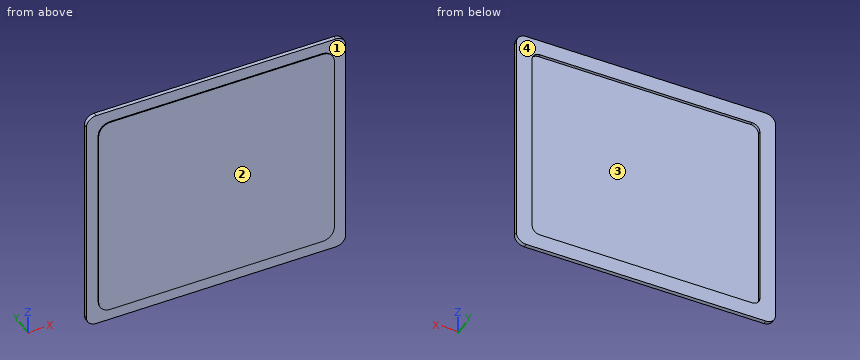
from build123d import *

# Parameters (mm, degrees)
RESSALTO_EXTRUS_O2_DEPTH = 10
RESSALTO_EXTRUS_O3_DEPTH = 2.5


with BuildPart() as part:
    # Esboço1 → Ressalto-extrusão2 (new body)
    with BuildSketch(Plane(origin=(0, 0, 0), x_dir=(1, 0, 0), z_dir=(0, 1, 0))):
        with BuildLine():
            Line((-305, -300), (305, -300))
            ThreePointArc((305, -300), (322.67766953, -292.67766953), (330, -275))
            Line((330, -275), (330, 275))
            ThreePointArc((330, 275), (322.67766953, 292.67766953), (305, 300))
            Line((305, 300), (-305, 300))
            ThreePointArc((-305, 300), (-322.67766953, 292.67766953), (-330, 275))
            Line((-330, 275), (-330, -275))
            ThreePointArc((-330, -275), (-322.67766953, -292.67766953), (-305, -300))
        make_face()
        with BuildLine():
            Line((270, -260), (-270, -260))
            ThreePointArc((-270, -260), (-284.142135624, -254.142135624), (-290, -240))
            Line((-290, -240), (-290, 240))
            ThreePointArc((-290, 240), (-284.142135624, 254.142135624), (-270, 260))
            Line((-270, 260), (270, 260))
            ThreePointArc((270, 260), (284.142135624, 254.142135624), (290, 240))
            Line((290, 240), (290, -240))
            ThreePointArc((290, -240), (284.142135624, -254.142135624), (270, -260))
        make_face(mode=Mode.SUBTRACT)
    extrude(amount=RESSALTO_EXTRUS_O2_DEPTH)

    # Esboço2 → Ressalto-extrusão3 (add, symmetric)
    with BuildSketch(Plane(origin=(0, 0, 0), x_dir=(1, 0, 0), z_dir=(0, 1, 0))):
        with BuildLine():
            Line((300, -240), (300, 240))
            ThreePointArc((300, 240), (291.213203436, 261.213203436), (270, 270))
            Line((270, 270), (-270, 270))
            ThreePointArc((-270, 270), (-291.213203436, 261.213203436), (-300, 240))
            Line((-300, 240), (-300, -240))
            ThreePointArc((-300, -240), (-291.213203436, -261.213203436), (-270, -270))
            Line((-270, -270), (270, -270))
            ThreePointArc((270, -270), (291.213203436, -261.213203436), (300, -240))
        make_face()
    extrude(amount=RESSALTO_EXTRUS_O3_DEPTH, both=True)


solid = part.part
For this review, take the finished solid that the model builds, in its own axes (mm). Face numbers are marked on the shaded views. A direction names the side the tool comes from. Coordinates: 2 decimals unless noted, no trailing zeros. Loops run counter-clockwise (first coordinate to the right, second up) from the corner with the lowest first, then second, coordinate; pieces in that order, holes last. Notation, with made-up numbers: (-32, 62.5) - (25, 62.5) arc R35 ccw to (25, 94.5) - close; hole circle Ø11 at (56.5, -38.75). An arc over 180 degrees is marked (long way). Use a Markdown table: item, result. Add a question column.
Item 1: Tool access review of the marked faces 1 and 2: name each direction out of +Z, -Z, +X, -X, +Y, -Y from which nothing blocks a thin tool from reaching the whole face with its end or side.
Item 2: We need section B-B (x = -45.5). Give the boundary of the cut face in (y, z).
Item 3: For line 1 (X direction, y = 5.25, z = -145); line 2 (Z direction, x = 10, y = 4.5); line 3 (Y direction, x = 5, z = -191.5), list the stretches that pass through material, from the lowest coordinate up.
Item 4: We need section C-C (z = -108). Give the boundary of the cut face in (x, y), and give its area (3 significant figures).
Item 5: Mouldability with a two-part tool opening along X and no side actions: class the marked faces 3 and 4 as pulls with the +X half, pulls with the -X half, needs draft (parallel to the pull), parting line crosses it, or undercut.
Item 6: We need section A-A (y = 6). Give the boundary of the cut face in (x, z).
Item 7: Insertion check: pin 1 Ø0.8 at (x, y) = (-117, -0.5) entering from +Z; pin 2 Ø6 at (x, z) = (-134.5, -118) entering from +Y; pin 3 Ø0.8 at (y, z) = (-1.5, 104.5) entering from -X; pin 4 Ø2 at (x, y) = (-37.5, -0.5) entering from -Z. Each pin has a flat end and moves straight along its axis. Give the tip position at first contact, or say it passes through.
Results list:
| question | item | result |
|---|---|---|
| 1 | face 1 | -Y |
| 1 | face 2 | +Z, -Z, +X, -X, -Y |
| 2 | outline | (-2.5, -270) - (0, -270) - (0, -300) - (10, -300) - (10, -260) - (2.5, -260) - (2.5, 260) - (10, 260) - (10, 300) - (0, 300) - (0, 270) - (-2.5, 270) - close |
| 3 | line 1 | x = -330 to -290, 290 to 330 |
| 3 | line 2 | z = -300 to -260, 260 to 300 |
| 3 | line 3 | y = -2.5 to 2.5 |
| 4 | outline | (-330, 0) - (-300, 0) - (-300, -2.5) - (300, -2.5) - (300, 0) - (330, 0) - (330, 10) - (290, 10) - (290, 2.5) - (-290, 2.5) - (-290, 10) - (-330, 10) - close |
| 4 | area | 3,750 mm^2 |
| 5 | face 3 | undercut |
| 5 | face 4 | needs draft |
| 6 | outline | (-330, -275) arc R25 ccw to (-305, -300) - (305, -300) arc R25 ccw to (330, -275) - (330, 275) arc R25 ccw to (305, 300) - (-305, 300) arc R25 ccw to (-330, 275) - close; hole (-290, -240) arc R20 ccw to (-270, -260) - (270, -260) arc R20 ccw to (290, -240) - (290, 240) arc R20 ccw to (270, 260) - (-270, 260) arc R20 ccw to (-290, 240) - close |
| 7 | pin 1 | stops at z = 270 |
| 7 | pin 2 | stops at y = 2.5 |
| 7 | pin 3 | stops at x = -300 |
| 7 | pin 4 | stops at z = -300 |
